from build123d import *

# Parameters (mm, degrees)
SKETCH1_R           = 127
BOSS_EXTRUDE1_DEPTH = 6.35
CUT_EXTRUDE1_DEPTH  = 7.35


with BuildPart() as part:
    # Sketch1 → Boss-Extrude1 (new body)
    with BuildSketch(Plane(origin=(0, 0, 0), x_dir=(1, 0, 0), z_dir=(0, 1, 0))):
        Circle(SKETCH1_R)
    extrude(amount=BOSS_EXTRUDE1_DEPTH)

    # Sketch2 → Cut-Extrude1 (cut, through all)
    with BuildSketch(Plane(origin=(0, 6.35, 0), x_dir=(1, 0, 0), z_dir=(0, 1, 0))):
        with BuildLine():
            Line((-60.237491978, 57.363810019), (-54.849338305, 51.975656347))
            ThreePointArc((-54.849338305, 51.975656347), (-51.975656347, 51.975656347), (-51.975656347, 54.849338305))
            Line((-51.975656347, 54.849338305), (-57.363810019, 60.237491978))
            ThreePointArc((-57.363810019, 60.237491978), (-60.237491978, 60.237491978), (-60.237491978, 57.363810019))
        make_face()
        with BuildLine():
            ThreePointArc((54.849338305, 51.975656347), (51.975656347, 51.975656347), (51.975656347, 54.849338305))
            Line((51.975656347, 54.849338305), (57.363810019, 60.237491978))
            ThreePointArc((57.363810019, 60.237491978), (60.237491978, 60.237491978), (60.237491978, 57.363810019))
            Line((60.237491978, 57.363810019), (54.849338305, 51.975656347))
        make_face()
        with BuildLine():
            ThreePointArc((66.703276385, 63.829594426), (63.829594426, 63.829594426), (63.829594426, 66.703276385))
            Line((63.829594426, 66.703276385), (69.217748099, 72.091430058))
            ThreePointArc((69.217748099, 72.091430058), (72.091430058, 72.091430058), (72.091430058, 69.217748099))
            Line((72.091430058, 69.217748099), (66.703276385, 63.829594426))
        make_face()
        with BuildLine():
            Line((60.237491978, -57.363810019), (54.849338305, -51.975656347))
            ThreePointArc((54.849338305, -51.975656347), (51.975656347, -51.975656347), (51.975656347, -54.849338305))
            Line((51.975656347, -54.849338305), (57.363810019, -60.237491978))
            ThreePointArc((57.363810019, -60.237491978), (60.237491978, -60.237491978), (60.237491978, -57.363810019))
        make_face()
        with BuildLine():
            Line((72.091430058, -69.217748099), (66.703276385, -63.829594426))
            ThreePointArc((66.703276385, -63.829594426), (63.829594426, -63.829594426), (63.829594426, -66.703276385))
            Line((63.829594426, -66.703276385), (69.217748099, -72.091430058))
            ThreePointArc((69.217748099, -72.091430058), (72.091430058, -72.091430058), (72.091430058, -69.217748099))
        make_face()
        with BuildLine():
            ThreePointArc((-54.849338305, -51.975656347), (-51.975656347, -51.975656347), (-51.975656347, -54.849338305))
            Line((-51.975656347, -54.849338305), (-57.363810019, -60.237491978))
            ThreePointArc((-57.363810019, -60.237491978), (-60.237491978, -60.237491978), (-60.237491978, -57.363810019))
            Line((-60.237491978, -57.363810019), (-54.849338305, -51.975656347))
        make_face()
        with BuildLine():
            ThreePointArc((-66.703276385, -63.829594426), (-63.829594426, -63.829594426), (-63.829594426, -66.703276385))
            Line((-63.829594426, -66.703276385), (-69.217748099, -72.091430058))
            ThreePointArc((-69.217748099, -72.091430058), (-72.091430058, -72.091430058), (-72.091430058, -69.217748099))
            Line((-72.091430058, -69.217748099), (-66.703276385, -63.829594426))
        make_face()
        with BuildLine():
            Line((-69.217748099, 72.091430058), (-63.829594426, 66.703276385))
            ThreePointArc((-63.829594426, 66.703276385), (-63.829594426, 63.829594426), (-66.703276385, 63.829594426))
            Line((-66.703276385, 63.829594426), (-72.091430058, 69.217748099))
            ThreePointArc((-72.091430058, 69.217748099), (-72.091430058, 72.091430058), (-69.217748099, 72.091430058))
        make_face()
    extrude(amount=-CUT_EXTRUDE1_DEPTH, mode=Mode.SUBTRACT)


solid = part.part
Work out the finished part from the listing and answer in its coordinate system (mm). Give positions to 0.01 mm unless a question says otherwise; leave off trailing zeros. Write each loop counter-clockwise with the first axis right and the second up, starting at its lowest first coordinate (ties: lowest second). Pieces come first, ordered by that corner, then holes.
Q1. The part is cut by section C-C on x = 106. Give the vertices of the cut face in (y, z), and give its area (3 significant figures).
Answer:
outline: (0, -69.95) - (6.35, -69.95) - (6.35, 69.95) - (0, 69.95) - close
area: 888 mm2
Q2. Given pin 1 (5 mm diameter, centred on x = -8.5, z = 92, fed in from -Y); pin 2 (1 mm diameter, centred on y = 4.5, z = 78, fed in from +X), each flat-ended and moving along its own axis, determine where each tip first touches the part or whether it passes through.
Answer:
pin 1: stops at y = 0
pin 2: stops at x = 100.61
Q3. The part is cut by section A-A on y = 2.75. State how many separate pieces and enclosed holes the cut face has, and give its area (3 significant figures).
Answer:
separate pieces: 1
enclosed holes: 8
area: 50,300 mm2
Q4. Straight lines are drawn through the part: L1, parallel to Z at x = -70, y = 5.25; L2, parallel to Z at x = 69.5, y = 6; L3, parallel to Z at x = 111.5, y = 1.75. For each, find the intervals that lie inside material, in ascending order.
Answer:
L1: z = -105.97 to -72.58, -67.13 to 67.13, 72.58 to 105.97
L2: z = -106.3 to -72.33, -66.63 to 66.63, 72.33 to 106.3
L3: z = -60.8 to 60.8
Q5. The part is cut by section B-B on x = -30.5. Give the vertices of the cut face in (y, z), and give its area (3 significant figures).
Answer:
outline: (0, -123.28) - (6.35, -123.28) - (6.35, 123.28) - (0, 123.28) - close
area: 1,570 mm2
